Autodesk Inventor part; units mm, degrees
ref_plane "YZ Plane" through (0, 0, 0) normal (1, 0, 0) x (0, 1, 0)
ref_plane "XZ Plane" through (0, 0, 0) normal (0, 1, 0) x (-1, 0, 0)
ref_plane "XY Plane" through (0, 0, 0) normal (0, 0, 1) x (1, 0, 0)
sketch "Sketch1" plane through (0, 0, 0) normal (0, 0, 1) x (1, 0, 0)
  arc A0 (0.5408, 16.1042) -> (0.5408, -9.1933) centre (-5.3897, 3.4555) ccw
  arc A1 (3.2365, 21.8536) -> (3.2365, -14.9427) centre (-5.3897, 3.4555) ccw
  arc A2 (-8.6245, 10.3548) -> (-12.2365, 0.111) centre (-5.3897, 3.4555) ccw
  line L0 (-11.3201, 16.1042) -> (-8.6245, 10.3548)
  line L1 (-5.3897, 3.4555) -> (3.2365, 21.8536) construction
  line L2 (-5.3897, 3.4555) -> (3.2365, -14.9427) construction
  line L3 (-5.3897, 3.4555) -> (14.9303, 3.4555) construction
  line L4 (-5.3897, 3.4555) -> (-14.0158, -14.9427) construction
  line L5 (-5.3897, 3.4555) -> (-14.0158, 21.8536) construction
  arc A3 (-8.6245, 10.3548) -> (-8.6245, -3.4438) centre (-5.3897, 3.4555) ccw
  line L6 (-8.6245, -3.4438) -> (-11.3201, -9.1933)
  line L7 (0.5408, 16.1042) -> (3.2365, 21.8536)
  line L8 (0.5408, -9.1933) -> (3.2365, -14.9427)
  line L9 (-19.3597, 3.4555) -> (-19.3597, -7.0739) construction
  point P0 (0, 0)
  dimension "d0" = 27.94
  dimension "d1" = 40.64
  dimension "d2" = 15.24
  dimension "d4" = 129.76
extrude "Extrusion1" add sketch "Sketch1" along normal blind 25.4
ref_plane "Work Plane1" through (-19.3597, 3.4555, 0) normal (-1, 0, 0) x (0, -1, 0)
sketch "Sketch2" plane through (-19.3597, 3.4555, 0) normal (-1, 0, 0) x (0, -1, 0)
  line L0 (-20.32, 0) -> (-20.32, 25.4)
  line L1 (20.32, 25.4) -> (-20.32, 25.4)
  line L2 (-20.32, 0) -> (20.32, 25.4)
  line L3 (-20.32, 25.4) -> (20.32, 0)
  line L4 (20.32, 0) -> (20.32, 25.4)
  circle A0 centre (0, 12.7) radius 8.89
  point P0 (3.4555, 0)
  point P1 (-18.3981, 25.4)
  point P2 (18.3981, 25.4)
  dimension "d7" = 17.78
extrude "Extrusion2" add sketch "Sketch2" along normal blind 127 contours A0 L3 L2 | L2 L3 A0 | A0 L2 L3 | L2 A0 L3
properties part number "golf2"
For this review, take the finished solid that the model builds, in its own axes (mm). A direction names the side the tool comes from. Give positions to 0.01 mm unless a question says otherwise; leave off trailing zeros. Loops run counter-clockwise (first coordinate to the right, second up) from the corner with the lowest first, then second, coordinate; pieces in that order, holes last. Notation, with made-up numbers: (36, -37) -> (78, -37) arc R17 cw to (78, -28) -> close; hole circle Ø11 at (22.25, -25.5). An arc over 180 degrees is marked (long way). One line per question, with ' | ' between items.
1) We need section D-D (z = 15). Write out the cut boundary in (x, y).
Resolved:
outline: (-146.36, -5.13) -> (-23.81, -5.13) arc R20.32 ccw to (3.24, -14.94) -> (0.54, -9.19) arc R13.97 cw to (-11.32, -9.19) -> (-8.62, -3.44) arc R7.62 cw to (-12.24, 0.11) arc R7.62 cw to (-8.62, 10.35) -> (-11.32, 16.1) arc R13.97 cw to (0.54, 16.1) -> (3.24, 21.85) arc R20.32 ccw to (-23.81, 12.04) -> (-146.36, 12.04) -> close
2) We need section B-B (y = 7). Write out the cut boundary in (x, z), plus the area to 3 significant figures.
Resolved:
outline: (-146.36, 4.55) -> (-25.4, 4.55) -> (-25.4, 0) -> (-12.14, 0) -> (-12.14, 25.4) -> (-25.4, 25.4) -> (-25.4, 20.85) -> (-146.36, 20.85) -> close | area: 2,310 mm2
3) The part is to be moulded in two halves that separate along X. For faces 4 (the cylindrical face through (-5.475, 17.425, 12.522)), 5 (the cylindrical face through (-84.151, -0.647, 20.587)), 6 (the flat face through (-9.953, -6.278, 12.522)), say which applies: +X half, -X half, draft (parallel to the pull), parting line (faces both ways), or undercut.
Resolved:
face 4: undercut | face 5: draft | face 6: +X half
4) To check wall thickness, follow probe 1 along X at (y, z) = (3, 14.25); probe 2 along Y at (x, z) = (-12, 24.25); probe 3 along Y at (x, z) = (-7.5, 17.75). State the ranges of each line that lie inside material, in increasing order.
Resolved:
probe 1: x = -146.36 to -13 | probe 2: y = -15.76 to -0.34, 7.25 to 22.67 | probe 3: y = -16.75 to -10.35, 17.27 to 23.67
5) Insertion check: pin 1 Ø5 at (x, z) = (-29, 17.5) entering from +Y; pin 2 Ø4 at (x, y) = (-107, 11.5) entering from -Z; pin 3 Ø1.5 at (x, y) = (-91.5, 5) entering from +Z; pin 4 Ø2 at (x, y) = (-35, 14) entering from +Z. Each pin has a flat end and moves straight along its axis. Give the tip position at first contact, or say it passes through.
Resolved:
pin 1: stops at y = 12.04 | pin 2: stops at z = 6.18 | pin 3: stops at z = 21.55 | pin 4: passes through
6) For faces 1 (the cylindrical face through (-5.304, -10.514, 12.522)), 2 (the flat face through (-15, 4, 0)), 3 (the flat face through (-9.99, 13.27, 12.52)), list the 3-axis set-ups (+Z, -Z, +X, -X, +Y, -Y) from which the entire face can be reached by the end or side of a thin tool; tool diameter is ignored.
Resolved:
face 1: +Z, -Z | face 2: -Z, +X, -X, +Y, -Y | face 3: +Z, -Z, +X
7) We need section C-C (x = -77.5). Write out the cut boundary in (y, z), plus the area to 3 significant figures.
Resolved:
outline: circle Ø17.78 at (3.46, 12.7) | area: 248 mm2
8) We need section A-A (z = 7.5). Write out the cut boundary in (x, y).
Resolved:
outline: (-146.36, -3.76) -> (-24.39, -3.76) arc R20.32 ccw to (3.24, -14.94) -> (0.54, -9.19) arc R13.97 cw to (-11.32, -9.19) -> (-8.62, -3.44) arc R7.62 cw to (-12.24, 0.11) arc R7.62 cw to (-8.62, 10.35) -> (-11.32, 16.1) arc R13.97 cw to (0.54, 16.1) -> (3.24, 21.85) arc R20.32 ccw to (-24.39, 10.67) -> (-146.36, 10.67) -> close
